The model under review builds one solid part; all positions refer to its coordinate system, in mm. Give positions to 0.01 mm unless a question says otherwise; leave off trailing zeros. Order: outer loops, then holes, each group sorted by start corner. A loop starts at its lowest first (then second) coordinate and runs counter-clockwise, first axis right, second up. Notation, with made-up numbers: (27.5, 3) -> (73.5, 3) arc R32 ccw to (73.5, 34) -> close; hole circle Ø7 at (-14, -16.5). An arc over 180 degrees is marked (long way). Use one line per item in the form item = value.
```python
from build123d import *

# Parameters (mm, degrees)
F0_R     = 3.175
F1_DEPTH = 3.048


with BuildPart() as f1:
    # F0 (on Front) → F1 (new body)
    with BuildSketch(Plane.XZ):
        with BuildLine():
            ThreePointArc((15.748631, 61.500946), (15.843376, 62.498478), (15.874999, 63.5))
            ThreePointArc((15.874999, 63.5), (15.843376, 64.501522), (15.748631, 65.499054))
            ThreePointArc((15.748631, 65.499054), (0.563144, 79.365008), (-15.567259, 66.610643))
            Line((-15.567259, 66.610643), (-15.853733, 64.321458))
            ThreePointArc((-15.853733, 64.321458), (-15.863991, 62.908862), (-15.748633, 61.500946))
            ThreePointArc((-15.748633, 61.500946), (0, 47.625), (15.748631, 61.500946))
        make_face()
        with Locations((-1e-06, 63.5)):
            Circle(F0_R, mode=Mode.SUBTRACT)
        with BuildLine():
            ThreePointArc((-15.567259, 66.610643), (0.563144, 79.365008), (15.748631, 65.499054))
            Line((15.748631, 65.499054), (9.521553, 114.556243))
            ThreePointArc((9.521553, 114.556243), (9.524138, 114.428133), (9.525, 114.3))
            ThreePointArc((9.525, 114.3), (-0.592526, 104.793448), (-9.451281, 115.482757))
            Line((-9.451281, 115.482757), (-15.567259, 66.610643))
        make_face()
        with Locations((-5.080221, 100.0252)):
            Circle(F0_R, mode=Mode.SUBTRACT)
        with BuildLine():
            Line((10.08135, 16.853859), (15.748631, 61.500946))
            ThreePointArc((15.748631, 61.500946), (0, 47.625), (-15.748633, 61.500946))
            Line((-15.748633, 61.500946), (-7.816068, -0.992133))
            ThreePointArc((-7.816068, -0.992133), (-0.497057, 7.86309), (7.878784, 0))
            ThreePointArc((7.878784, 0), (6.238207, -4.812486), (1.9997, -7.62079))
            Line((1.9997, -7.62079), (44.390741, -7.937279))
            ThreePointArc((44.390741, -7.937279), (36.512537, 0.024387), (44.439515, 7.937493))
            Line((44.439515, 7.937493), (17.978767, 7.90254))
            ThreePointArc((17.978767, 7.90254), (12.006638, 10.593011), (10.08135, 16.853859))
        make_face()
        with BuildLine():
            Line((-15.853733, 64.321458), (-15.567259, 66.610643))
            ThreePointArc((-15.567259, 66.610643), (-15.752135, 65.471261), (-15.853733, 64.321458))
        make_face()
        with BuildLine():
            ThreePointArc((9.525, 114.3), (9.524138, 114.428133), (9.521553, 114.556243))
            ThreePointArc((9.521553, 114.556243), (0.464587, 123.813663), (-9.451281, 115.482757))
            ThreePointArc((-9.451281, 115.482757), (-0.592526, 104.793448), (9.525, 114.3))
        make_face()
        with Locations((0, 114.3)):
            Circle(F0_R, mode=Mode.SUBTRACT)
        with BuildLine():
            ThreePointArc((7.878784, 0), (-0.497057, 7.86309), (-7.816068, -0.992133))
            ThreePointArc((-7.816068, -0.992133), (-4.409343, -6.52939), (1.9997, -7.62079))
            ThreePointArc((1.9997, -7.62079), (6.238207, -4.812486), (7.878784, 0))
        make_face()
        Circle(F0_R, mode=Mode.SUBTRACT)
        with BuildLine():
            ThreePointArc((52.3875, 0), (50.058952, 5.616366), (44.439515, 7.937493))
            ThreePointArc((44.439515, 7.937493), (36.512537, 0.024387), (44.390741, -7.937279))
            ThreePointArc((44.390741, -7.937279), (50.04167, -5.633572), (52.3875, 0))
        make_face()
        with Locations((44.45, 0)):
            Circle(F0_R, mode=Mode.SUBTRACT)
    extrude(amount=F1_DEPTH)


solid = f1.part
```
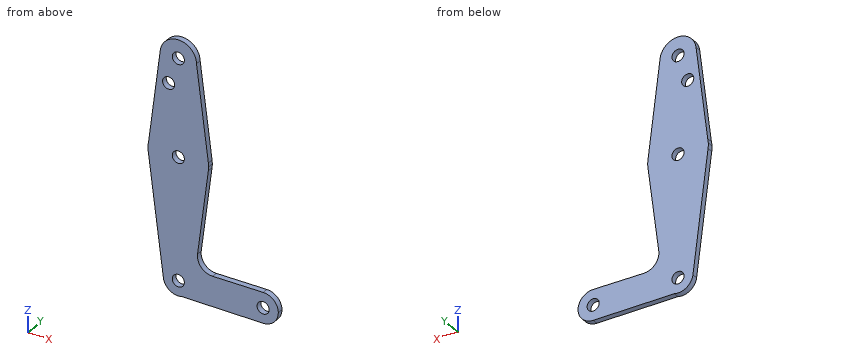
1. Add section C-C on z = 56.5. Give the boundary of the cut face in (x, y), then the cut area to 3 significant figures.
Values:
outline = (-15.11, -3.05) -> (15.11, -3.05) -> (15.11, 0) -> (-15.11, 0) -> close
area = 92.1 mm^2
2. Add section B-B on y = -0.95. Count the separate pieces of the cut face and the enclosed holes in it, then the cut area to 3 significant figures.
Values:
separate_pieces = 1
enclosed_holes = 5
area = 3,600 mm^2
3. Add section A-A on x = 0. Give the boundary of the cut face in (y, z) (3 decimals).
Values:
outline = (-3.048, -7.879) -> (0, -7.879) -> (0, -3.175) -> (-3.048, -3.175) -> close; (-3.048, 3.175) -> (0, 3.175) -> (0, 60.325) -> (-3.048, 60.325) -> close; (-3.048, 66.675) -> (0, 66.675) -> (0, 111.125) -> (-3.048, 111.125) -> close; (-3.048, 117.475) -> (0, 117.475) -> (0, 123.825) -> (-3.048, 123.825) -> close
4. For pin 1 Ø5.5 at (x, z) = (0, 0) entering from +Y; pin 2 Ø1 at (y, z) = (-2.5, 68) entering from +X; pin 3 Ø1.5 at (x, y) = (41, -2) entering from +Z; pin 4 Ø1.5 at (y, z) = (-2, 35) entering from -X, all flat-tipped, find the tip position at first contact; note any pin that passes through.
Values:
pin_1 = through
pin_2 = 15.49
pin_3 = 7.93
pin_4 = -12.48
5. Add section D-D on z = 74. Give the boundary of the cut face in (x, y), then the cut area to 3 significant figures.
Values:
outline = (-14.64, -3.05) -> (14.67, -3.05) -> (14.67, 0) -> (-14.64, 0) -> close
area = 89.3 mm^2
6. For L1, parallel to Z at x = 0, y = -2.8 (3 decimals); L2, parallel to X at y = -1.5, z = 2.5; L3, parallel to Z at x = 40.5, y = -1.05, list the stretches that pass through material, from the lowest coordinate up.
Values:
L1 = -7.879 to -3.175, 3.175 to 60.325, 66.675 to 111.125, 117.475 to 123.825
L2 = -8.26 to -1.96, 1.96 to 42.49, 46.41 to 51.98
L3 = -7.91 to 7.93
